Can you work these out from the model? Positions are in its coordinate system, mm. A direction names the side the tool comes from. Coordinates: 2 decimals unless noted, no trailing zeros. Loops run counter-clockwise (first coordinate to the right, second up) from the corner with the lowest first, then second, coordinate; pieces in that order, holes last. Notation, with made-up numbers: (67.25, 76.5) -> (75.25, 76.5) arc R16 ccw to (75.25, 103.5) -> close; hole circle Ø3 at (82.5, 5). An arc over 180 degrees is marked (long way). Use one line per item in the form item = value. Start each with the question number.
(1) Imagine slicing it at A-A (y = 10). List the corners of the cut face in (x, z) for me.
(2) Imagine slicing it at C-C (x = -54.5). List the corners of the cut face in (y, z) for me.
(3) Imagine slicing it at B-B (z = 7). List the corners of the cut face in (x, y) for me.
(4) Imagine slicing it at D-D (y = 0). List the corners of the cut face in (x, z) for me.
(5) I'm going to push flat-ended pins straight in: pin 1 (12 mm diameter, centred on x = -29.5, z = 12, fed in from -Y); pin 2 (12 mm diameter, centred on x = -39, y = -12, fed in from -Z); pin 3 (4 mm diameter, centred on x = -43, z = 4, fed in from -Y). Where does each tip first touch, or does it pass through?
(6) On a 3-axis mill with a long thin cutter (end or side, diameter ignored), from which of +Z, -Z, +X, -X, +Y, -Y can I reach the whole of each face in a straight line? I mean faces 1 (the cylindrical face through (-34.603, 8.799, -4.93)), 2 (the flat face through (-38, -10, 20)), 3 (the cylindrical face through (-34.603, -8.799, 14.93)). Say none if no direction works.
(7) I need wall thicknesses on line 1 (Z direction, x = -49.5, y = -8); line 2 (X direction, y = 2, z = 8); line 3 (X direction, y = -11, z = 6.5). Which ranges of each line are inside material? Lowest first, please. Write a range as [from, to].
```python
from build123d import *

# Parameters (mm, degrees)
F0_R     = 20
F1_DEPTH = 10
F2_R     = 4
F3_DEPTH = 10
F4_R     = 4
F5_DEPTH = 10


with BuildPart() as f1:
    # F0 (on Top) → F1 (new body)
    with BuildSketch(Plane.XY):
        with Locations((-38.417947, 0)):
            Circle(F0_R)
    extrude(amount=F1_DEPTH)

    # F2 (on face) → F3 (join)
    with BuildSketch(Plane(origin=(0, 0, 0), x_dir=(1, 0, 0), z_dir=(0, 0, -1))):
        with Locations((-38.417947, -10)):
            Circle(F2_R)
    extrude(amount=F3_DEPTH)

    # F4 (on face) → F5 (join)
    with BuildSketch(Plane.XY.offset(10)):
        with Locations((-38.417947, -10)):
            Circle(F4_R)
    extrude(amount=F5_DEPTH)


solid = f1.part
```
Worked out:
q1.outline = (-55.74, 0) -> (-42.42, 0) -> (-42.42, -10) -> (-34.42, -10) -> (-34.42, 0) -> (-21.1, 0) -> (-21.1, 10) -> (-55.74, 10) -> close
q2.outline = (-11.89, 0) -> (11.89, 0) -> (11.89, 10) -> (-11.89, 10) -> close
q3.outline = circle Ø40 at (-38.42, 0)
q4.outline = (-58.42, 0) -> (-18.42, 0) -> (-18.42, 10) -> (-58.42, 10) -> close
q5.pin_1 = -19.73
q5.pin_2 = 0
q5.pin_3 = -19.83
q6.face_1 = -Z
q6.face_2 = +Z, +X, -X, +Y, -Y
q6.face_3 = +Z
q7.line_1 = [0, 10]
q7.line_2 = [-58.32, -18.52]
q7.line_3 = [-55.12, -21.71]
